from build123d import *

# Parameters (mm, degrees)
SKETCH_1_R             = 20
EXTRUDE_1_DEPTH        = 5
SKETCH_2_R             = 1.525
CUT_EXTRUDE_1_DEPTH    = 5
SKETCH_3_R             = 7
EXTRUDE_2_DEPTH        = 4
SKETCH_4_R             = 5
EXTRUDE_3_DEPTH        = 15
CHAMFER_2_SIZE         = 1.05
CUT_EXTRUDE_2_DEPTH    = 15
SKETCH_7_R             = 3
EXTRUDE_4_DEPTH        = 10
SKETCH_8_R             = 20
SKETCH_8_R_2           = 7
CUT_EXTRUDE_3_DEPTH    = 1
SKETCH_9_R             = 20
SKETCH_9_R_2           = 1.525
EXTRUDE_5_DEPTH        = 3
SKETCH_10_R            = 20
SKETCH_10_R_2          = 7
CUT_EXTRUDE_4_DEPTH    = 3
SKETCH_11_R            = 3
EXTRUDE_6_DEPTH        = 1
HOLE_WIZARD_M3_1_D     = 2.5
HOLE_WIZARD_M3_1_DEPTH = 5
HOLE_WIZARD_M3_1_TIP   = 0.751075774
CHAMFER_3_SIZE         = 0.5
HOLE_WIZARD_M5_1_D     = 4.2
CHAMFER_4_SIZE         = 1


with BuildPart() as part:
    # 草图1 → 凸台-拉伸1 (new body)
    with BuildSketch(Plane.XY):
        Circle(SKETCH_1_R)
    extrude(amount=EXTRUDE_1_DEPTH)

    # 草图2 → 切除-拉伸1 (cut)
    with BuildSketch(Plane.XY.offset(5)):
        with Locations((13.5, 0)):
            Circle(SKETCH_2_R)
        with Locations((6.75, -11.691342951)):
            Circle(SKETCH_2_R)
        with Locations((-6.75, -11.691342951)):
            Circle(SKETCH_2_R)
        with Locations((-13.5, 0)):
            Circle(SKETCH_2_R)
        with Locations((-6.75, 11.691342951)):
            Circle(SKETCH_2_R)
        with Locations((6.75, 11.691342951)):
            Circle(SKETCH_2_R)
    extrude(amount=-CUT_EXTRUDE_1_DEPTH, mode=Mode.SUBTRACT)

    # 草图3 → 凸台-拉伸2 (add)
    with BuildSketch(Plane.XY.offset(5)):
        Circle(SKETCH_3_R)
    extrude(amount=EXTRUDE_2_DEPTH)

    # 草图4 → 凸台-拉伸3 (add)
    with BuildSketch(Plane.XY.offset(9)):
        Circle(SKETCH_4_R)
    extrude(amount=EXTRUDE_3_DEPTH)

    # 倒角2
    chamfer_2_edges = [part.edges().sort_by_distance(p)[0] for p in [
        (-7, 0, 9),
    ]]
    chamfer(chamfer_2_edges, length=CHAMFER_2_SIZE)

    # 草图6 → 切除-拉伸2 (cut)
    with BuildSketch(Plane.XY.offset(24)):
        with BuildLine():
            Line((-3, -4), (3, -4))
            ThreePointArc((3, -4), (0, -5), (-3, -4))
        make_face()
    extrude(amount=-CUT_EXTRUDE_2_DEPTH, mode=Mode.SUBTRACT)

    # 草图7 → 凸台-拉伸4 (add)
    with BuildSketch(Plane.XY.offset(24)):
        Circle(SKETCH_7_R)
    extrude(amount=EXTRUDE_4_DEPTH)

    # 草图8 → 切除-拉伸3 (cut)
    with BuildSketch(Plane.XY.offset(5)):
        Circle(SKETCH_8_R)
        Circle(SKETCH_8_R_2, mode=Mode.SUBTRACT)
    extrude(amount=-CUT_EXTRUDE_3_DEPTH, mode=Mode.SUBTRACT)

    # 草图9 → 凸台-拉伸5 (add)
    with BuildSketch(Plane(origin=(0, 0, 0), x_dir=(-1, 0, 0), z_dir=(0, 0, -1))):
        Circle(SKETCH_9_R)
        with Locations((6.75, 11.691342951)):
            Circle(SKETCH_9_R_2, mode=Mode.SUBTRACT)
        with Locations((13.5, 0)):
            Circle(SKETCH_9_R_2, mode=Mode.SUBTRACT)
        with Locations((6.75, -11.691342951)):
            Circle(SKETCH_9_R_2, mode=Mode.SUBTRACT)
        with Locations((-6.75, -11.691342951)):
            Circle(SKETCH_9_R_2, mode=Mode.SUBTRACT)
        with Locations((-13.5, 0)):
            Circle(SKETCH_9_R_2, mode=Mode.SUBTRACT)
        with Locations((-6.75, 11.691342951)):
            Circle(SKETCH_9_R_2, mode=Mode.SUBTRACT)
    extrude(amount=EXTRUDE_5_DEPTH)

    # 草图10 → 切除-拉伸4 (cut)
    with BuildSketch(Plane.XY.offset(4)):
        Circle(SKETCH_10_R)
        Circle(SKETCH_10_R_2, mode=Mode.SUBTRACT)
    extrude(amount=-CUT_EXTRUDE_4_DEPTH, mode=Mode.SUBTRACT)

    # 草图11 → 凸台-拉伸6 (add)
    with BuildSketch(Plane.XY.offset(34)):
        Circle(SKETCH_11_R)
    extrude(amount=EXTRUDE_6_DEPTH)

    # M3 螺纹孔1
    with Locations(Plane.XY.offset(35)):
        with Locations((0, 0)):
            Hole(HOLE_WIZARD_M3_1_D / 2, depth=HOLE_WIZARD_M3_1_DEPTH)
            with Locations((0, 0, -(HOLE_WIZARD_M3_1_DEPTH + HOLE_WIZARD_M3_1_TIP / 2))):  # 118° drill point
                Cone(0, HOLE_WIZARD_M3_1_D / 2, HOLE_WIZARD_M3_1_TIP, mode=Mode.SUBTRACT)

    # 倒角3
    chamfer_3_edges = [part.edges().sort_by_distance(p)[0] for p in [
        (-20, 0, 1),
        (20, 0, -3),
    ]]
    chamfer(chamfer_3_edges, length=CHAMFER_3_SIZE)

    # M5 螺纹孔1 (through all)
    with Locations(Plane(origin=(0, -4, 20.1), x_dir=(0, 0, -1), z_dir=(0, -1, 0))):
        with Locations((0, 0)):
            Hole(HOLE_WIZARD_M5_1_D / 2)

    # 倒角4
    chamfer_4_edges = [part.edges().sort_by_distance(p)[0] for p in [
        (-7, 0, 1),
    ]]
    chamfer(chamfer_4_edges, length=CHAMFER_4_SIZE)

    # 草图22 → 旋转2 (revolve)
    with BuildSketch(Plane(origin=(0, 0, 0), x_dir=(1, 0, 0), z_dir=(0, 1, 0))):
        Polygon((6.5, -6.833333333), (10, -1), (6.5, -1), align=None)
    revolve(axis=Axis((0, 0, 0), (0, 0, 1)))


solid = part.part
Model file for the job. Use its own axes, mm. A direction names the side the tool comes from. Give positions to 0.01 mm unless a question says otherwise; leave off trailing zeros. Order: outer loops, then holes, each group sorted by start corner. A loop starts at its lowest first (then second) coordinate and runs counter-clockwise, first axis right, second up. Notation, with made-up numbers: (75.25, -28) - (110.25, -28) arc R20 cw to (110.25, -6) - close; hole circle Ø9 at (59, 41). An arc over 180 degrees is marked (long way). Write item = value, one per line. Start each with the question number.
1. Which spindle directions (+Z, -Z, +X, -X, +Y, -Y) get a long thin tool onto all of the face, cutting with end or side? Do faces 1 (the flat face through (0, -4, 17)), 2 (the flat face through (2, 3, 24)), 3 (the cylindrical face through (0.631, 0.565, 22.103)). Say none if no direction does.
2. Cut at A-A, the plane z = 20.1. List the corners of the cut face in (x, y), and give its area (3 significant figures).
3. Cut at D-D, the plane z = 4.5. List the corners of the cut face in (x, y).
4. Cut at B-B, the plane z = 25. List the corners of the cut face in (x, y).
5. Two-plate mould, pull along Y, no slides. Class faces 4 (the cylindrical face through (0.27, -1.22, 32.47)), 5 (the flat face through (-9, 5, 1)), 6 (the cylindrical face through (-3, 0, 29)): pulls with the +Y half, pulls with the -Y half, needs draft (parallel to the pull), parting line crosses it, or undercut.
6. Probe line 1 along X through (y, z) = (0, -0.6) (3 decimals); line 2 along Y through (x, z) = (0, 32); line 3 along Y through (x, z) = (-6.75, -0.55). List the from-to ranges inside material, lowest first.
7. Drop flat-ended pins along their axis: P1, Ø2, axis at x = -1, y = -11.5, coming from the +Z side; P2, Ø3, axis at x = -6, z = 15.5, coming from the -Y side; P3, Ø5, axis at y = -0.5, z = 27.5, coming from the +X side. Give the stop position or say it passes through.
8. Cut at C-C, the plane y = 11. State how many separate pieces and enclosed holes the cut face has, and give its area (3 significant figures).
Taken from the geometry:
q1.face_1 = +Z, +X, -X, -Y
q1.face_2 = +Z
q1.face_3 = +Y, -Y
q2.outline = (-3, -4) - (-2.1, -4) - (-2.1, 4.54) arc R5 ccw to start; (2.1, -4) - (3, -4) arc R5 ccw to (2.1, 4.54) - close
q2.area = 37.3 mm²
q3.outline = circle Ø15.8 at (0, 0)
q4.outline = circle Ø6 at (0, 0)
q5.face_4 = undercut
q5.face_5 = needs draft
q5.face_6 = parting line crosses it
q6.line_1 = -20 to -15.025, -11.975 to 11.975, 15.025 to 20
q6.line_2 = -3 to -1.25, 1.25 to 3
q6.line_3 = -18.83 to -13.22, -10.17 to 10.17, 13.22 to 18.83
q7.P1 = 1
q7.P2 = -2.18
q7.P3 = 3
q8.separate_pieces = 3
q8.enclosed_holes = 0
q8.area = 111 mm²
